Autodesk Inventor part; units mm, degrees
ref_plane "Work Plane1" through (0, 0, 10.45) normal (0, 0, 1) x (1, 0, 0)
ref_plane "Work Plane2" through (0, 0, 4.75) normal (0, 0, 1) x (1, 0, 0)
ref_plane "YZ Plane" through (0, 0, 0) normal (1, 0, 0) x (0, 1, 0)
sketch "Sketch1" plane through (0, 0, 0) normal (0, 0, 1) x (1, 0, 0)
  line L0 (-11.9, 0) -> (11.9, 0) construction
  line L1 (0, -13.7409) -> (0, 13.7409) construction
  line L2 (0, 9.815) -> (8.5, 4.9075)
  line L3 (8.5, 4.9075) -> (8.5, -4.9075)
  line L4 (8.5, -4.9075) -> (0, -9.815)
  line L5 (0, -9.815) -> (-8.5, -4.9075)
  line L6 (-8.5, -4.9075) -> (-8.5, 4.9075)
  line L7 (-8.5, 4.9075) -> (0, 9.815)
  point P0 (0, 0)
  point P1 (0, 0)
  dimension "d67" = 17
extrude "Выдавливание1" add sketch "Sketch1" along normal blind 9.5
ref_plane "Work Plane1" through (0, 0, 10.45) normal (0, 0, 1) x (1, 0, 0)
ref_plane "Work Plane2" through (0, 0, 4.75) normal (0, 0, 1) x (1, 0, 0)
sketch "Sketch2" plane through (0, 0, 9.5) normal (0, 0, 1) x (1, 0, 0)
  point P0 (0, 0)
hole "Отверстие1" at (0, 0, 9.5) direction (0, 0, -1) diameter 8.376 end through all
sketch "Sketch3" plane through (0, 0, 0) normal (1, 0, 0) x (0, 1, 0)
  line L0 (-4.9075, 9.5) -> (4.9075, 9.5) construction
  line L1 (4.9075, 9.5) -> (9.815, 9.5) construction
  line L2 (-9.815, 9.5) -> (-4.9075, 9.5) construction
  line L3 (-4.188, 0) -> (-4.188, 9.5) construction
  line L4 (4.9075, 0) -> (4.9075, 9.5) construction
  line L5 (0, -1.9) -> (0, 11.4) construction
  line L6 (-5, 9.5) -> (0, 4.5)
  line L7 (0, 4.5) -> (0, 9.5)
  line L8 (0, 9.5) -> (-5, 9.5)
  line L9 (5, 9.5) -> (0, 4.5)
  line L10 (0, 9.5) -> (5, 9.5)
  point P0 (0, 0)
  dimension "d57" = 45
  dimension "d58" = 10
revolve "Вращение1" cut sketch "Sketch3" angle 360 about axis through (0, 0, -10) along (0, 0, 1) contours L8 L7 L6
sketch "Sketch4" plane through (0, 0, 0) normal (1, 0, 0) x (0, 1, 0)
  line L0 (-7.25, 9.5) -> (-12.25, 6.6132)
  line L1 (-12.25, 6.6132) -> (-12.25, 9.5)
  line L2 (0, -1.9) -> (0, 11.4) construction
  line L3 (-7.25, 9.5) -> (-12.25, 9.5)
  line L4 (7.25, 9.5) -> (12.25, 6.6132)
  line L5 (12.25, 6.6132) -> (12.25, 9.5)
  line L6 (7.25, 9.5) -> (12.25, 9.5)
  point P0 (0, 0)
  dimension "d11" = 30
  dimension "d12" = 14.5
  dimension "d13" = 24.5
  dimension "d60" = 9.5
revolve "Вращение2" cut sketch "Sketch4" angle 360 about axis through (0, 0, -10) along (0, 0, 1) contours L0 L1 L3
mirror "Симметричное отображение1" about plane through (0, 0, 4.75) normal (0, 0, 1) of "Вращение2"
sketch "Sketch5" plane through (0, 0, 0) normal (1, 0, 0) x (0, 1, 0)
  line L0 (4.188, 0) -> (-4.188, 0) construction
  line L1 (0, -1.9) -> (0, 11.4) construction
  line L2 (-5, 0) -> (0, 5)
  line L3 (0, 0) -> (-5, 0)
  line L4 (-4.188, 0) -> (4.188, 0) construction
  line L5 (2.5, 0) -> (-2.5, 0) construction
  line L6 (5, 0) -> (0, 5)
  line L7 (0, 0) -> (5, 0)
  line L8 (0, 5) -> (0, 0)
  point P0 (-1.2295, 3.4)
  point P1 (1.2295, 3.4)
  point P2 (-4.188, 9.5)
  dimension "d54" = 45
  dimension "d55" = 10
revolve "Вращение3" cut sketch "Sketch5" angle 360 about axis through (0, 0, -10) along (0, 0, 1) contours L2 L8 L3
equation "\"d67\" = S_"
equation "\"d1\" = m_"
equation "\"d12\" = dw"
equation "\"d13\" = dw + da"
equation "\"d55\" = da"
equation "\"d58\" = da"
equation "\"S_\" = 17"
equation "\"e\" = 18.48"
equation "\"da\" = 10"
equation "\"dw\" = 14.5"
equation "\"m_\" = 9.5"
equation "\"d15\" = 0.1 * m_"
properties part number "ГайкаM10ГОСТ ISO 4034-2014" material "Сталь, мягкая"
The model under review builds one solid part; all positions refer to its coordinate system, in mm. Coordinates: 2 decimals unless noted, no trailing zeros. Order: outer loops, then holes, each group sorted by start corner. A loop starts at its lowest first (then second) coordinate and runs counter-clockwise, first axis right, second up. Notation, with made-up numbers: M 62.5,22.5 L 91.5,22.5 A33 cw 91.5,59.5 Z; hole C 69,86 d9. An arc over 180 degrees is marked long. One line per question, with ' | ' between items.
(1) For probe 1 along X at (y, z) = (0, 8.5); probe 2 along Y at (x, z) = (1.5, 5.5); probe 3 along Y at (x, z) = (1.75, 5), list the stretches that pass through material, from the lowest coordinate up. Write a range as from..to.
Geometry results:
probe 1: x = -8.5..-4.19, 4.19..8.5 | probe 2: y = -8.95..-3.91, 3.91..8.95 | probe 3: y = -8.8..-3.8, 3.8..8.8
(2) Add section B-B, the plane z = 2.25. Write out the cut boundary in (x, y) (1 decimal), then the cut area to 3 significant figures.
Geometry results:
outline: M -8.5,-4.9 L 0,-9.8 L 8.5,-4.9 L 8.5,4.9 L 0,9.8 L -8.5,4.9 Z; hole C 0,0 d8.4 | area: 195 mm²
(3) Add section A-A, the plane y = 0. Write out the cut boundary in (x, z), then the cut area to 3 significant figures.
Geometry results:
outline: M -8.5,0.72 L -7.25,0 L -5,0 L -4.19,0.81 L -4.19,8.69 L -5,9.5 L -7.25,9.5 L -8.5,8.78 Z; M 4.19,0.81 L 5,0 L 7.25,0 L 8.5,0.72 L 8.5,8.78 L 7.25,9.5 L 5,9.5 L 4.19,8.69 Z | area: 78.8 mm²
(4) The part is to be moulded in two halves that separate along Y. For faces 1 (the face through (-4.31, 7.327, 4.694)), 2 (the face through (-8.5, 0, 5)), 3 (the face through (-2.83, 3.087, 4.695)), 4 (the face through (4.31, -7.327, 4.694)), say which applies: +Y half, -Y half, draft (parallel to the pull), parting line (faces both ways), or undercut.
Geometry results:
face 1: +Y half | face 2: draft | face 3: undercut | face 4: -Y half
